The listing builds one solid part. Answer for the finished solid, in the listing's coordinates (mm). A direction names the side the tool comes from. Give positions to 0.01 mm unless a question says otherwise; leave off trailing zeros. Order: outer loops, then holes, each group sorted by start corner. A loop starts at its lowest first (then second) coordinate and runs counter-clockwise, first axis right, second up. Notation, with made-up numbers: (83.5, -29.5) -> (107.5, -29.5) arc R31 cw to (107.5, 5.5) -> close; hole circle Ø3 at (-7.5, 7.25). An arc over 180 degrees is marked (long way). One line per question, with ' | ' between items. Start each with the question number.
```python
from build123d import *

# Parameters (mm, degrees)
SKETCH11_W                     = 355
SKETCH11_H                     = 300
SKETCH11_R                     = 15
BOSS_EXTRUDE2_DEPTH            = 10
CBORE_START                    = 5
CBORE_FOR_M5_SHCS1_OUTLINE_R   = 5
CBORE_FOR_M5_SHCS1_DEPTH       = 5
CBORE_FOR_M5_SHCS1_2_OUTLINE_R = 2.75
CBORE_FOR_M5_SHCS1_2_DEPTH     = 5
FILLET1_R                      = 75


# Read off the part's stored shape, not the designer's step: CBORE for M5 SHCS1
with BuildPart() as part:
    # Sketch11 → Boss-Extrude2 (new body)
    with BuildSketch(Plane(origin=(0, 0, 0), x_dir=(1, 0, 0), z_dir=(0, 1, 0))):
        Rectangle(SKETCH11_W, SKETCH11_H)
        with Locations(Location((67.5, -125, 0), (0, 0, 270))):
            Circle(SKETCH11_R, mode=Mode.SUBTRACT)
        with Locations(Location((67.5, 125, 0), (0, 0, 270))):
            Circle(SKETCH11_R, mode=Mode.SUBTRACT)
    extrude(amount=BOSS_EXTRUDE2_DEPTH)

    # CBORE for M5 SHCS1 outline → CBORE for M5 SHCS1 (cut)
    with BuildSketch(Plane(origin=(0, 0, 0), x_dir=(1, 0, 0), z_dir=(0, 1, 0)).offset(CBORE_START)):
        with Locations((137.5, 100)):
            Circle(CBORE_FOR_M5_SHCS1_OUTLINE_R)
        with Locations((-137.5, -100)):
            Circle(CBORE_FOR_M5_SHCS1_OUTLINE_R)
        with Locations((-137.5, 100)):
            Circle(CBORE_FOR_M5_SHCS1_OUTLINE_R)
        with Locations((137.5, -100)):
            Circle(CBORE_FOR_M5_SHCS1_OUTLINE_R)
    extrude(amount=CBORE_FOR_M5_SHCS1_DEPTH, mode=Mode.SUBTRACT)

    # CBORE for M5 SHCS1 2 outline → CBORE for M5 SHCS1 2 (cut)
    with BuildSketch(Plane(origin=(0, 0, 0), x_dir=(1, 0, 0), z_dir=(0, 1, 0))):
        with Locations((137.5, 100)):
            Circle(CBORE_FOR_M5_SHCS1_2_OUTLINE_R)
        with Locations((-137.5, -100)):
            Circle(CBORE_FOR_M5_SHCS1_2_OUTLINE_R)
        with Locations((-137.5, 100)):
            Circle(CBORE_FOR_M5_SHCS1_2_OUTLINE_R)
        with Locations((137.5, -100)):
            Circle(CBORE_FOR_M5_SHCS1_2_OUTLINE_R)
    extrude(amount=CBORE_FOR_M5_SHCS1_2_DEPTH, mode=Mode.SUBTRACT)

    # Fillet1
    fillet1_edges = [part.edges().sort_by_distance(p)[0] for p in [
        (177.5, 5, -150),
        (177.5, 5, 150),
        (-177.5, 5, 150),
        (-177.5, 5, -150),
    ]]
    fillet(fillet1_edges, radius=FILLET1_R)


solid = part.part
```
(1) For faces 4 (the face through (-156.11, 5.07, 127.45)), 5 (the face through (136.42, 7.46, 104.88)), determine the directions among +Z, -Z, +X, -X, +Y, -Y from which every point of the face is accessible in a straight line to the end or side of a thin tool.
(2) The part is cut by section A-A on y = 1.5. Determine the outline of the cut face in (x, z), plus the area to 3 significant figures.
(3) Consider line 1 (X direction, y = 1.5, z = 100); line 2 (Z direction, x = -137.5, y = 8.4); line 3 (Z direction, x = 137.5, y = 2.35). Determine where each line is inside the solid, lowest interval first.
(4) The part is cut by section B-B on x = 67.5. Determine the outline of the cut face in (y, z).
(5) Given P1, Ø11, axis at x = -136.5, z = 99, coming from the +Y side; P2, Ø6, axis at x = 137.5, z = -100, coming from the +Y side; P3, Ø18, axis at x = 67.5, z = -125, coming from the +Y side; P4, Ø4, axis at y = 7, z = 86.5, coming from the +X side, each flat-ended and moving along its own axis, determine where each tip first touches the part or whether it passes through.
(6) The part is cut by section C-C on z = -125. Determine the outline of the cut face in (x, y), plus the area to 3 significant figures.
(7) Determine the mould class of faces 1 (the face through (-141.5, 7.5, -97)), 2 (the face through (-2, 0, -2)), 3 (the face through (-156.11, 5.07, -127.45)) for opening direction X: pulls with the +X half, pulls with the -X half, needs draft (parallel to the pull), parting line crosses it, or undercut.
Result sheet:
1) face 4: +Z, -X, +Y, -Y | face 5: +Y
2) outline: (-177.5, -75) arc R75 ccw to (-102.5, -150) -> (102.5, -150) arc R75 ccw to (177.5, -75) -> (177.5, 75) arc R75 ccw to (102.5, 150) -> (-102.5, 150) arc R75 ccw to (-177.5, 75) -> close; hole circle Ø5.5 at (-137.5, -100); hole circle Ø5.5 at (-137.5, 100); hole circle Ø30 at (67.5, -125); hole circle Ø30 at (67.5, 125); hole circle Ø5.5 at (137.5, -100); hole circle Ø5.5 at (137.5, 100) | area: 100,000 mm^2
3) line 1: x = -173.21 to -140.25, -134.75 to 134.75, 140.25 to 173.21 | line 2: z = -141.33 to -105, -95 to 95, 105 to 141.33 | line 3: z = -141.33 to -102.75, -97.25 to 97.25, 102.75 to 141.33
4) outline: (0, -150) -> (10, -150) -> (10, -140) -> (0, -140) -> close; (0, -110) -> (10, -110) -> (10, 110) -> (0, 110) -> close; (0, 140) -> (10, 140) -> (10, 150) -> (0, 150) -> close
5) P1: stops at y = 10 | P2: stops at y = 5 | P3: passes through | P4: stops at x = 176.9
6) outline: (-158.4, 0) -> (52.5, 0) -> (52.5, 10) -> (-158.4, 10) -> close; (82.5, 0) -> (158.4, 0) -> (158.4, 10) -> (82.5, 10) -> close | area: 2,870 mm^2
7) face 1: undercut | face 2: needs draft | face 3: pulls with the -X half
